Autodesk Inventor part; units mm, degrees
ref_plane "YZ Plane" through (0, 0, 0) normal (1, 0, 0) x (0, 1, 0)
ref_plane "XZ Plane" through (0, 0, 0) normal (0, 1, 0) x (-1, 0, 0)
ref_plane "XY Plane" through (0, 0, 0) normal (0, 0, 1) x (1, 0, 0)
sketch "Sketch1" plane through (0, 0, 0) normal (0, 1, 0) x (-1, 0, 0)
  line L0 (0, 0) -> (0, -16.5)
  line L1 (0, -16.5) -> (0, 16.5)
  circle A0 centre (0, -14.5) radius 2
  circle A1 centre (0, 14.5) radius 2
  line L2 (3.5, 0) -> (2.5, 0)
  line L3 (2, 14.5) -> (2.5, 2.4495)
  line L4 (2.5, -2.4495) -> (1.9983, -14.5826)
  line L5 (-1.9983, -14.5826) -> (-2.5, -2.4495)
  line L6 (-2.5299, 2.4186) -> (-1.9983, 14.5826)
  arc A2 (2.5, -2.4495) -> (2.5, 2.4495) centre (0, 0) ccw
  arc A3 (-2.5299, 2.4186) -> (-2.5, -2.4495) centre (0, 0) ccw
  dimension "d2" = 33
  dimension "d3" = 4
  dimension "d4" = 4
  dimension "d5" = 2
  dimension "d6" = 2
  dimension "d7" = 1
extrude "Extrusion1" add sketch "Sketch1" along normal blind 1.5
sketch "Sketch2" plane through (0, 1.5, 0) normal (0, 1, 0) x (1, 0, 0)
  circle A0 centre (0, 0) radius 3.5
extrude "Extrusion2" add sketch "Sketch2" along normal blind 2
sketch "Sketch3" plane through (0, 3.5, 0) normal (0, 1, 0) x (1, 0, 0)
  circle A0 centre (0, 0) radius 2
  dimension "d13" = 4
extrude "Extrusion3" cut sketch "Sketch3" against normal blind 2
sketch "Sketch4" plane through (0, 1.5, 0) normal (0, 1, 0) x (1, 0, 0)
  circle A0 centre (0, 5.3571) radius 0.375
  circle A1 centre (0, 7.2143) radius 0.375
  circle A2 centre (0, 9.0714) radius 0.375
  circle A3 centre (0, 10.9286) radius 0.375
  circle A4 centre (0, 12.7857) radius 0.375
  circle A5 centre (0, 14.6429) radius 0.375
  arc A6 (2.5, 2.4495) -> (-2.5, 2.4495) centre (0, 0) ccw
  dimension "d16" = 0.75
  dimension "d17" = 0.75
  dimension "d18" = 0.75
  dimension "d19" = 0.75
  dimension "d20" = 0.75
  dimension "d21" = 0.75
  dimension "d22" = 1.8571
  dimension "d23" = 5.3571
  dimension "d24" = 1.8571
  dimension "d25" = 1.8571
  dimension "d26" = 1.8571
  dimension "d27" = 1.8571
extrude "Extrusion4" cut sketch "Sketch4" against normal blind 2
mirror "Mirror1" about plane through (0, 0, 0) normal (0, 0, 1) of "Extrusion4"
properties part number "Micro Servo 9g Arm"
Read the model definition and answer for the solid it produces. Units are mm, in the model's axes. A direction names the side the tool comes from. Coordinates: 2 decimals unless noted, no trailing zeros. Loops run counter-clockwise (first coordinate to the right, second up) from the corner with the lowest first, then second, coordinate; pieces in that order, holes last. Notation, with made-up numbers: (75.25, 74) -> (99.25, 74) arc R18 ccw to (99.25, 99) -> close; hole circle Ø11 at (-11.75, 18). An arc over 180 degrees is marked (long way). Return JSON: item names as keys, results as strings.
Item 1: Find the intervals of material crossed by probe 1 along X at (y, z) = (2.2, 0); probe 2 along Y at (x, z) = (-2, -7.5); probe 3 along X at (y, z) = (0.8, 5.5), in increasing order.
Answers:
{"probe 1": "x = -3.5 to -2, 2 to 3.5", "probe 2": "y = 0 to 1.5", "probe 3": "x = -2.37 to -0.35, 0.35 to 2.4"}
Item 2: For faces 4 (the flat face through (2.246, 0.74, -8.601)), 5 (the cylindrical face through (0, 3, 2)), determine the directions among +Z, -Z, +X, -X, +Y, -Y from which every point of the face is accessible in a straight line to the end or side of a thin tool.
Answers:
{"face 4": "-Z, +X, +Y, -Y", "face 5": "+Y"}
Item 3: Find section B-B (z = 0). Determine the outline of the cut face in (x, y).
Answers:
{"outline": "(-3.5, 0) -> (3.5, 0) -> (3.5, 3.5) -> (2, 3.5) -> (2, 1.5) -> (-2, 1.5) -> (-2, 3.5) -> (-3.5, 3.5) -> close"}
Item 4: For a pull along Z with two mould halves and no side action, classify faces 1 (the cylindrical face through (-0.08, 0.74, -16.5)), 2 (the flat face through (0, 1.5, 0)), 3 (the flat face through (0, 0, 0)) as +Z half, -Z half, draft (parallel to the pull), parting line (faces both ways), or undercut.
Answers:
{"face 1": "-Z half", "face 2": "undercut", "face 3": "draft"}
Item 5: Find section D-D (x = 1.5). Determine the outline of the cut face in (y, z).
Answers:
{"outline": "(0, -15.82) -> (1.5, -15.82) -> (1.5, -3.16) -> (3.5, -3.16) -> (3.5, -1.32) -> (1.5, -1.32) -> (1.5, 1.32) -> (3.5, 1.32) -> (3.5, 3.16) -> (1.5, 3.16) -> (1.5, 15.82) -> (0, 15.82) -> close"}
Item 6: Find section A-A (y = 1.1). Count the separate pieces of the cut face and the enclosed holes in it, plus the area to 3 significant figures.
Answers:
{"separate pieces": "1", "enclosed holes": "12", "area": "147 mm2"}
Item 7: Flat-ended cylindrical pins translate along their axes: P1, Ø1.5, axis at x = -1, z = -6, coming from the +Y side; P2, Ø2, axis at x = 2, y = 2, coming from the +Z side; P3, Ø2, axis at x = -2.5, y = 0.5, coming from the -Z side. Find the tip coordinate at first contact, or state that the pin passes through.
Answers:
{"P1": "stops at y = 1.5", "P2": "stops at z = 16.15", "P3": "stops at z = -15.82"}
